For this review, use the dimensioned drawing (mm, ordinates from the lowest corner) and the shaded views. A direction names the side the tool comes from. Coordinates: 2 decimals unless noted, no trailing zeros. Loops run counter-clockwise (first coordinate to the right, second up) from the corner with the lowest first, then second, coordinate; pieces in that order, holes last. Notation, with made-up numbers: (-11, 50.5) -> (25, 50.5) arc R9 cw to (25, 62.5) -> close; hole circle Ø5 at (18, 63.25). An arc over 180 degrees is marked (long way). Answer as a JSON object with one key per item and string values.
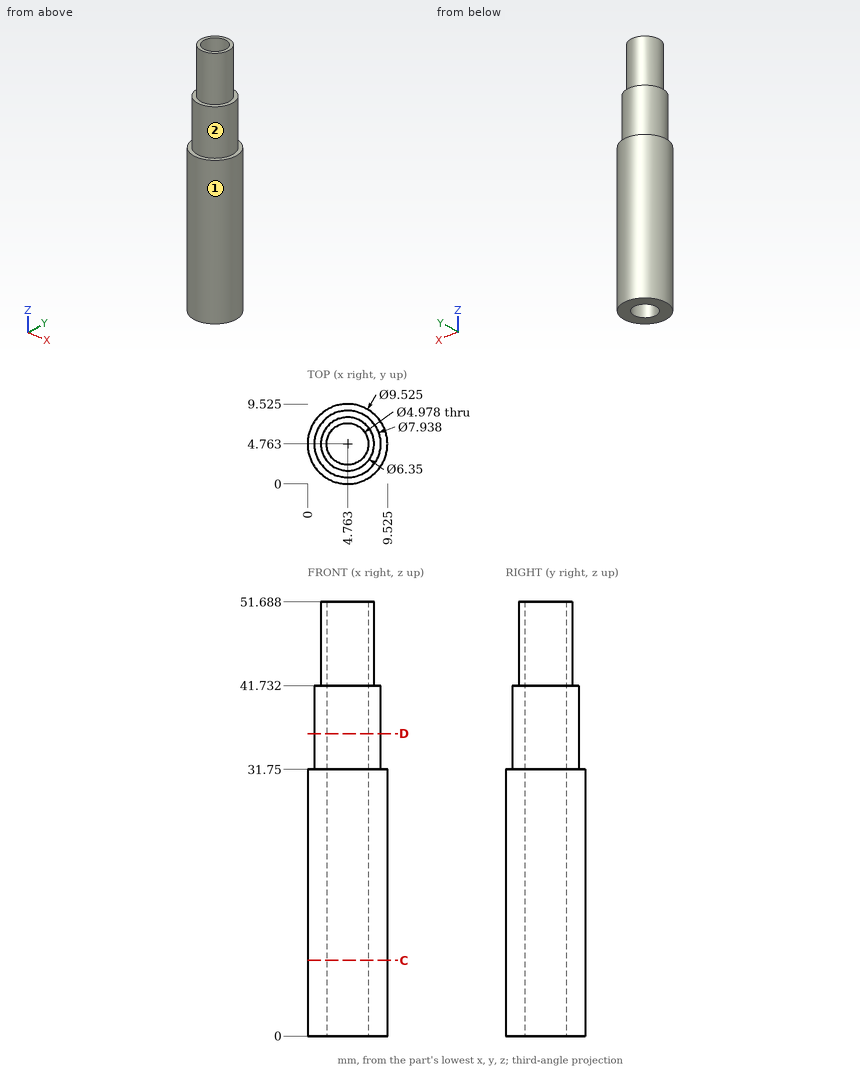
1) Clearance check with flat-ended pins moving along their axes: pin 1 Ø4.5 at (x, y) = (4.76, 4.76) entering from +Z; pin 2 Ø1.5 at (x, y) = (8.5, 7.5) entering from +Z; pin 3 Ø5 at (x, z) = (2.5, 38) entering from -Y; pin 4 Ø3 at (x, z) = (2, 43.5) entering from +Y (1 decimal). State where each tip first meets the part, or that it passes through.
Completed:
{"pin 1": "through", "pin 2": "z = 41.73", "pin 3": "y = 0.79", "pin 4": "y = 7.7"}
2) Add section C-C, the plane z = 9. Give the boundary of the cut face in (x, y) (1 decimal).
Completed:
{"outline": "circle Ø9.5 at (4.8, 4.8); hole circle Ø5 at (4.8, 4.8)"}
3) For the marked faces 1 and 2, list the 3-axis set-ups (+Z, -Z, +X, -X, +Y, -Y) from which the entire face can be reached by the end or side of a thin tool; tool diameter is ignored.
Completed:
{"face 1": "+Z, -Z", "face 2": "+Z"}
4) Add section D-D, the plane z = 36. Give the boundary of the cut face in (x, y).
Completed:
{"outline": "circle Ø7.94 at (4.76, 4.76); hole circle Ø4.98 at (4.76, 4.76)"}
5) Wall thickness on probe 1 along Y at (x, z) = (4.75, 37.5); probe 2 along Y at (x, z) = (5.25, 9.5) (1 decimal); probe 3 along X at (y, z) = (3.75, 36.5) (1 decimal): over which ranges is each line inside the solid? List them lowest first.
Completed:
{"probe 1": "0.79 to 2.27, 7.25 to 8.73", "probe 2": "0 to 2.3, 7.2 to 9.5", "probe 3": "0.9 to 2.5, 7 to 8.6"}
